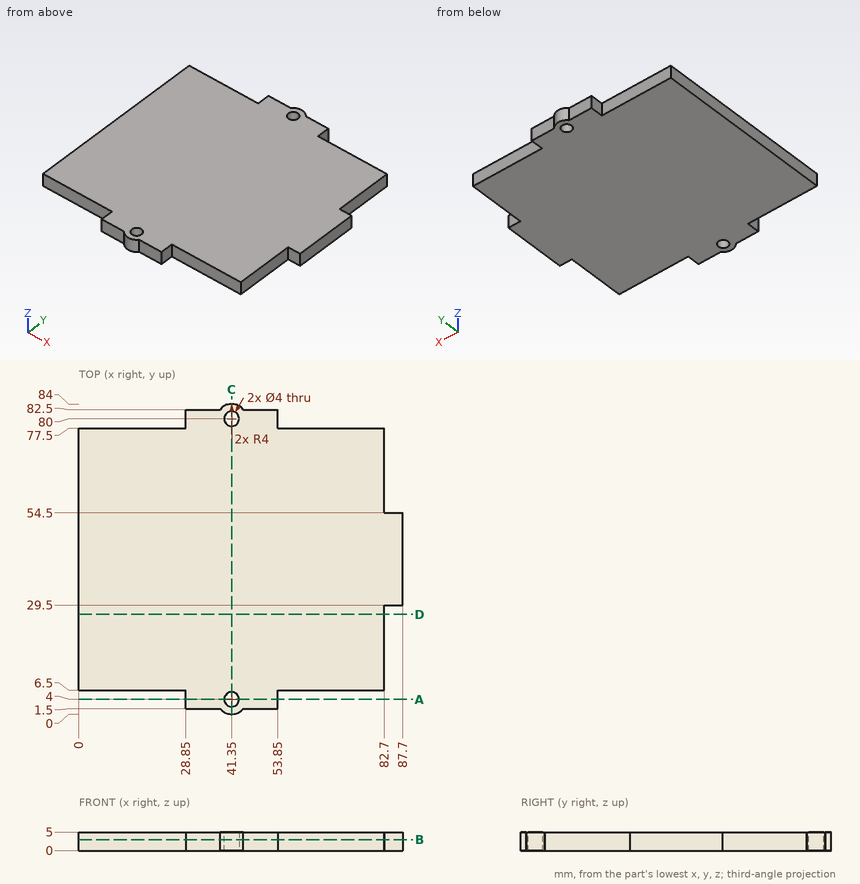
Drawing for the job (mm, zero at the part's lowest x, y, z). Give positions to 0.01 mm unless a question says otherwise; leave off trailing zeros. Loops run counter-clockwise (first coordinate to the right, second up) from the corner with the lowest first, then second, coordinate; pieces in that order, holes last.
1) Drop flat-ended pins along their axis: P1, Ø2.5, axis at x = 35.5, z = 3, coming from the -Y side; P2, Ø2, axis at x = 71.5, z = 1.5, coming from the +Y side; P3, Ø2.5, axis at y = 5, z = 3.5, coming from the +X side. Give the stop position or say it passes through.
Values follow:
P1: stops at y = 1.5
P2: stops at y = 77.5
P3: stops at x = 53.85
2) Probe line 1 along Y through (x, z) = (41.35, 2.1); line 2 along X through (y, z) = (80, 2.3); line 3 along Y through (x, z) = (64.5, 4.3). List the from-to ranges inside material, lowest first.
Values follow:
line 1: y = 0 to 2, 6 to 78, 82 to 84
line 2: x = 28.85 to 39.35, 43.35 to 53.85
line 3: y = 6.5 to 77.5
3) Band-saw the part on A-A on y = 4. List the corners of the cut face in (x, z).
Values follow:
outline: (28.85, 0) - (39.35, 0) - (39.35, 5) - (28.85, 5) - close; (43.35, 0) - (53.85, 0) - (53.85, 5) - (43.35, 5) - close
4) Band-saw the part on B-B on z = 3. List the corners of the cut face in (x, y), then the cut area to 3 significant figures.
Values follow:
outline: (0, 6.5) - (28.85, 6.5) - (28.85, 1.5) - (38.23, 1.5) arc R4 ccw to (44.47, 1.5) - (53.85, 1.5) - (53.85, 6.5) - (82.7, 6.5) - (82.7, 29.5) - (87.7, 29.5) - (87.7, 54.5) - (82.7, 54.5) - (82.7, 77.5) - (53.85, 77.5) - (53.85, 82.5) - (44.47, 82.5) arc R4 ccw to (38.23, 82.5) - (28.85, 82.5) - (28.85, 77.5) - (0, 77.5) - close; hole circle Ø4 at (41.35, 4); hole circle Ø4 at (41.35, 80)
area: 6,230 mm2
5) Band-saw the part on C-C on x = 41.35. List the corners of the cut face in (y, z).
Values follow:
outline: (0, 0) - (2, 0) - (2, 5) - (0, 5) - close; (6, 0) - (78, 0) - (78, 5) - (6, 5) - close; (82, 0) - (84, 0) - (84, 5) - (82, 5) - close
6) Band-saw the part on D-D on y = 27. List the corners of the cut face in (x, z).
Values follow:
outline: (0, 0) - (82.7, 0) - (82.7, 5) - (0, 5) - close
